The listing builds one solid part. Answer for the finished solid, in the listing's coordinates (mm). A direction names the side the tool comes from. Give positions to 0.01 mm unless a question says otherwise; leave off trailing zeros. Loops run counter-clockwise (first coordinate to the right, second up) from the corner with the lowest first, then second, coordinate; pieces in that order, holes last. Notation, with made-up numbers: M 25,-2 L 84,-2 A24 cw 84,10 Z; hole C 45.5,-31.75 d11. An arc over 180 degrees is marked long. Return JSON: item names as keys, results as strings.
from build123d import *

# Parameters (mm, degrees)
SKETCH_1_R          = 7.5
EXTRUDE_1_DEPTH     = 80
SKETCH_2_R          = 1.65
CUT_EXTRUDE_1_DEPTH = 10


with BuildPart() as part:
    # ｽｹｯﾁ1 → ﾎﾞｽ - 押し出し1 (new body)
    with BuildSketch(Plane.XY):
        Circle(SKETCH_1_R)
    extrude(amount=EXTRUDE_1_DEPTH)

    # ｽｹｯﾁ2 → ｶｯﾄ - 押し出し1 (cut)
    with BuildSketch(Plane.XY.offset(80)):
        Circle(SKETCH_2_R)
    cut_extrude_1 = extrude(amount=-CUT_EXTRUDE_1_DEPTH, mode=Mode.SUBTRACT)

    # ﾐﾗｰ1: ｶｯﾄ - 押し出し1 across plane
    add(cut_extrude_1.mirror(Plane.XY.offset(40)), mode=Mode.SUBTRACT)


solid = part.part
(1) Straight lines are drawn through the part: line 1 along Y through (x, z) = (0, 7.75); line 2 along X through (y, z) = (6.75, 17); line 3 along Y through (x, z) = (5.25, 69.5). For each, find the intervals that lie inside material, in ascending order.
Values follow:
{"line 1": "-7.5 to -1.65, 1.65 to 7.5", "line 2": "-3.27 to 3.27", "line 3": "-5.36 to 5.36"}
(2) A tool of negligible diameter and unlimited length cuts with its end or side. For faces 1 (the cylindrical face through (-1.216, 1.115, 4.93)), 2 (the cylindrical face through (-1.216, 1.115, 75.07)), 3 (the flat face through (0, 2, 80)), from which of +Z, -Z, +X, -X, +Y, -Y can it reach the whole face along a straight path? Write none if from no direction.
Values follow:
{"face 1": "-Z", "face 2": "+Z", "face 3": "+Z, +X, -X, +Y, -Y"}
(3) Determine the mould class of faces 4 (the flat face through (0, 0, 70)), 5 (the cylindrical face through (-7.493, 0.33, 39.44)), 6 (the flat face through (0, 0, 10)), 7 (the flat face through (0, 2, 0)) for opening direction Y: released by +Y, released by -Y, zero draft, split by the parting line, or undercut.
Values follow:
{"face 4": "undercut", "face 5": "split by the parting line", "face 6": "undercut", "face 7": "zero draft"}
(4) The part is cut by section A-A (x = 0). Determine the outline of the cut face in (y, z).
Values follow:
{"outline": "M -7.5,0 L -1.65,0 L -1.65,10 L 1.65,10 L 1.65,0 L 7.5,0 L 7.5,80 L 1.65,80 L 1.65,70 L -1.65,70 L -1.65,80 L -7.5,80 Z"}
(5) The part is cut by section C-C (z = 75). Determine the outline of the cut face in (x, y), and give its area (3 significant figures).
Values follow:
{"outline": "C 0,0 d15; hole C 0,0 d3.3", "area": "168 mm²"}
(6) The part is cut by section D-D (z = 64.5). Determine the outline of the cut face in (x, y), and give its area (3 significant figures).
Values follow:
{"outline": "C 0,0 d15", "area": "177 mm²"}
(7) Given pin 1 (2.5 mm diameter, centred on x = -1, y = 0.5, fed in from -Z); pin 2 (1 mm diameter, centred on y = -6, z = 34, fed in from +X); pin 3 (2.5 mm diameter, centred on x = 0, y = 0, fed in from -Z); pin 4 (1.5 mm diameter, centred on y = -1.5, z = 33, fed in from -X), each flat-ended and moving along its own axis, determine where each tip first touches the part or whether it passes through.
Values follow:
{"pin 1": "z = 0", "pin 2": "x = 5.1", "pin 3": "z = 10", "pin 4": "x = -7.46"}
